The figure shows three views and two pictorial views of one solid part (mm, origin at its lowest corner). Answer the questions. Coordinates: 2 decimals unless noted, no trailing zeros. Order: outer loops, then holes, each group sorted by start corner. A loop starts at its lowest first (then second) coordinate and runs counter-clockwise, first axis right, second up. Notation, with made-up numbers: (35, 87) -> (82, 87) arc R29 ccw to (82, 122) -> close; hole circle Ø10 at (-7.75, 86). An arc over 180 degrees is marked (long way). Write item = value, one per line. Start each with the question number.
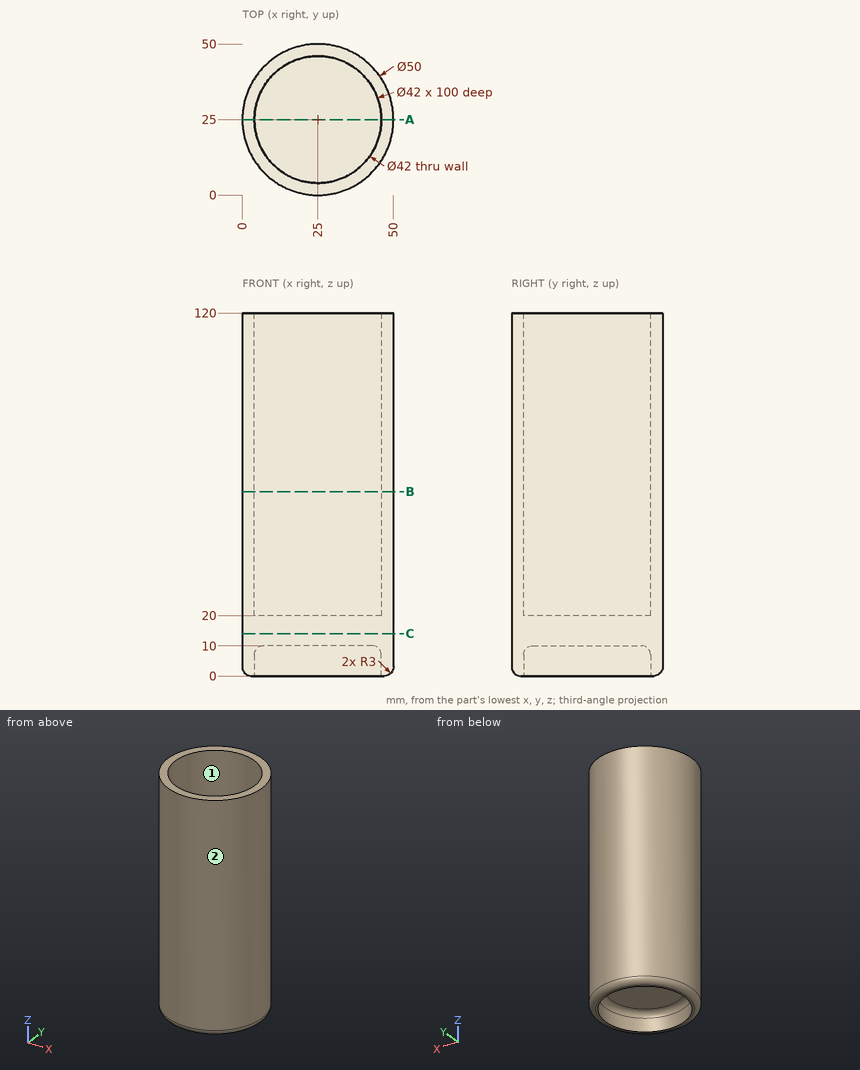
Item 1: Section A-A, the plane y = 25 is taken. Give the vertices of the cut face in (x, z).
Item 2: Consider probe 1 along Y at (x, z) = (25, 74); probe 2 along X at (y, z) = (6.5, 75); probe 3 along Y at (x, z) = (40.5, 21). Determine where each line is inside the solid, lowest interval first.
Item 3: For a pull along Y with two mould halves and no side action, classify the marked faces 1 and 2 as pulls with the +Y half, pulls with the -Y half, needs draft (parallel to the pull), parting line crosses it, or undercut.
Item 4: Section B-B, the plane z = 61 is taken. Give the vertices of the cut face in (x, y), then the cut area to 3 significant figures.
Item 5: Section C-C, the plane z = 14 is taken. Give the vertices of the cut face in (x, y).
Item 6: Each of these flat-tipped pins is pushed along its axis until it touches: pin 1 (4 mm diameter, centred on x = 32, z = 77.5, fed in from +Y); pin 2 (1.5 mm diameter, centred on x = 21.5, z = 39.5, fed in from +Y); pin 3 (5 mm diameter, centred on x = 20, y = 27, fed in from +Z). Where does it stop, or does it pass through?
A:
q1.outline = (0, 3) arc R3 ccw to (3, 0) -> (4, 0) -> (4, 7) arc R3 cw to (7, 10) -> (43, 10) arc R3 cw to (46, 7) -> (46, 0) -> (47, 0) arc R3 ccw to (50, 3) -> (50, 120) -> (46, 120) -> (46, 20) -> (4, 20) -> (4, 120) -> (0, 120) -> close
q2.probe_1 = 0 to 4, 46 to 50
q2.probe_2 = 8.18 to 15.06, 34.94 to 41.82
q2.probe_3 = 5.38 to 10.83, 39.17 to 44.62
q3.face_1 = undercut
q3.face_2 = parting line crosses it
q4.outline = circle Ø50 at (25, 25); hole circle Ø42 at (25, 25)
q4.area = 578 mm^2
q5.outline = circle Ø50 at (25, 25)
q6.pin_1 = 49.49
q6.pin_2 = 49.85
q6.pin_3 = 20
